Input: dimensioned drawing with shaded views. Units: mm. Origin: part minimum x, y, z. A direction names the side the tool comes from. Round coordinates to 2 decimals unless told otherwise and drop trailing zeros. Write each loop counter-clockwise with the first axis right and the second up, starting at its lowest first coordinate (ties: lowest second). Pieces come first, ordered by that corner, then holes. Notation, with made-up numbers: M 2.25,65.25 L 59.25,65.25 A18 cw 59.25,72.25 Z; hole C -30.75,69 d9. An arc over 180 degrees is marked long. Answer as CSV lines item,"result". Start each with the question number.
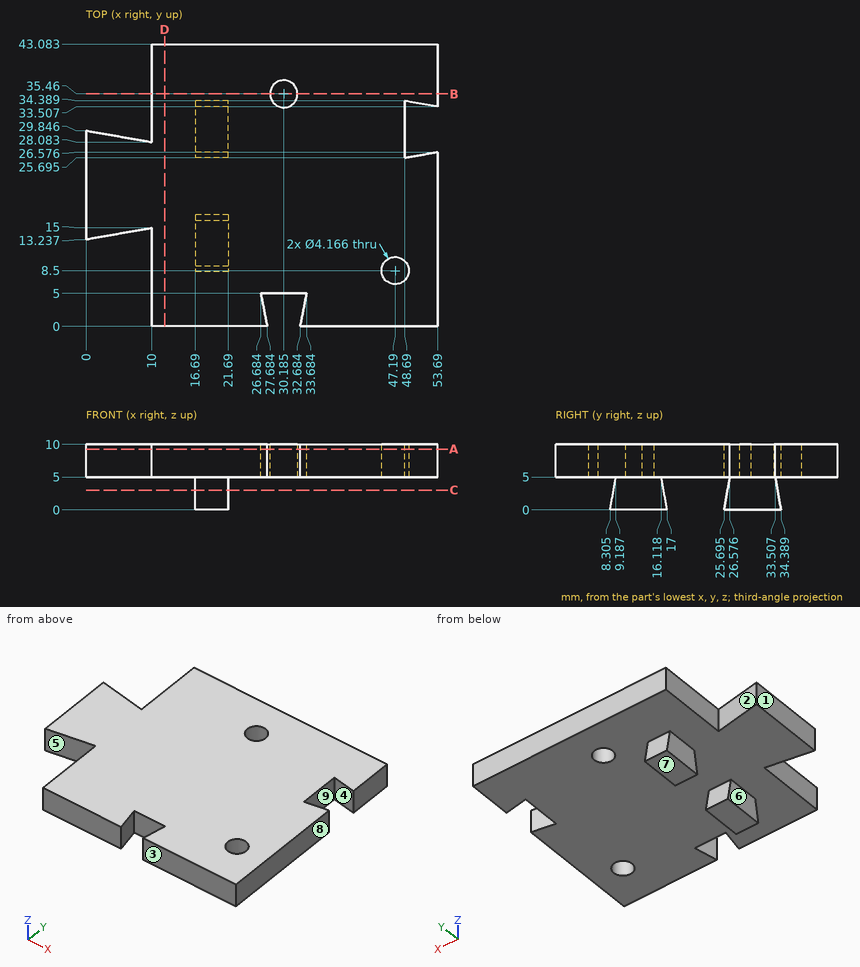
Item 1: Cut plane A-A, the plane z = 9.25. Return loops of the section in (x, y) (1 decimal), plus the area to 3 significant figures.
Item 2: Line query: line 1 (Z direction, x = 47, y = 15); line 2 (X direction, y = 29.5, z = 1.75); line 3 (Y direction, x = 4, z = 6.5). Output: solid intervals per line, ascending. Write a range as [from, to].
Item 3: Access query for the marked faces 5, 6, 7, 8 and 9. Directions: +Z, -Z, +X, -X, +Y, -Y. A direction counts if a zero-diameter tool reaches every point of the face in a straight line with its end or side. Return the directions, or none.
Item 4: Cut plane D-D, the plane x = 12. Return loops of the section in (y, z).
Item 5: Cut plane B-B, the plane y = 35.46. Return loops of the section in (x, z), plus the area to 3 significant figures.
Item 6: Pin query (flat end, axial travel): pin 1 Ø1 at (x, z) = (5.5, 8) entering from +Y (1 decimal); pin 2 Ø1.5 at (y, z) = (10.5, 2) entering from -X; pin 3 Ø5 at (x, y) = (18.5, 7.5) entering from -Z; pin 4 Ø2.5 at (y, z) = (35, 7.5) entering from -X. Return the tip coordinate at first contact, or that it passes through.
Item 7: Draft query along Y for the marked faces 1, 2, 3 and 4. Return one class per face: +Y half, -Y half, draft (parallel to the pull), parting line (faces both ways), or undercut.
Item 8: Cut plane C-C, the plane z = 3. Return loops of the section in (x, y) (1 decimal).
Results list:
1,outline,"M 0,13.2 L 10,15 L 10,0 L 27.7,0 L 26.7,5 L 33.7,5 L 32.7,0 L 53.7,0 L 53.7,26.6 L 48.7,25.7 L 48.7,34.4 L 53.7,33.5 L 53.7,43.1 L 10,43.1 L 10,28.1 L 0,29.8 Z; hole C 30.2,35.5 d4.2; hole C 47.2,8.5 d4.2"
1,area,"1,930 mm²"
2,line 1,"[5, 10]"
2,line 2,"[16.69, 21.69]"
2,line 3,"[13.94, 29.14]"
3,face 5,"+Z, -Z, -Y"
3,face 6,"-Z, -X, +Y, -Y"
3,face 7,"-Z, +X, -X, +Y, -Y"
3,face 8,"+Z, -Z, +X, +Y, -Y"
3,face 9,"+Z, -Z"
4,outline,"M 0,5 L 43.08,5 L 43.08,10 L 0,10 Z"
5,outline,"M 10,5 L 28.1,5 L 28.1,10 L 10,10 Z; M 32.27,5 L 53.69,5 L 53.69,10 L 32.27,10 Z"
5,area,"198 mm²"
6,pin 1,"y = 29"
6,pin 2,"x = 16.69"
6,pin 3,"z = 0"
6,pin 4,"x = 10"
7,face 1,"draft"
7,face 2,"+Y half"
7,face 3,"-Y half"
7,face 4,"undercut"
8,outline,"M 16.7,8.8 L 21.7,8.8 L 21.7,16.5 L 16.7,16.5 Z; M 16.7,26.2 L 21.7,26.2 L 21.7,33.9 L 16.7,33.9 Z"
